Here's how the part is built. I have some questions about the finished solid (model axes, mm). A direction names the side the tool comes from. Give positions to 0.01 mm unless a question says otherwise; leave off trailing zeros. Order: outer loops, then holes, each group sorted by start corner. A loop starts at its lowest first (then second) coordinate and runs counter-clockwise, first axis right, second up. Notation, with made-up numbers: (-37.5, -31.75) -> (12.5, -31.75) arc R20 ccw to (12.5, -12.75) -> close; hole circle Ø8 at (6, -31.5). An arc over 180 degrees is marked (long way). Write each question's results on one line, items separated by ' | '. Start each with the question number.
Q1. Imagine slicing it at B-B, the plane z = 5.5. Please give me the cut outline in (x, y).
Q2. Imagine slicing it at A-A, the plane y = -28. Please give me the cut outline in (x, z), then the cut area to 3 significant figures.
Q3. I need wall thicknesses on line 1 along X through (y, z) = (-43, 24); line 2 along Z through (x, y) = (-29, -39); line 3 along Y through (x, z) = (-0.5, 44). Which ranges of each line are inside material? Lowest first, please. Write a range as [from, to].
Q4. Thinking about a two-plate mould opening in X: for faces 1 (the face through (35, 29, 30)), 2 (the face through (92.171, 0, 52)), 3 (the face through (53, 20, 70)), which applies, pulls with the +X half, pulls with the -X half, needs draft (parallel to the pull), parting line crosses it, or undercut?
Q5. I'm going to push flat-ended pins straight in: pin 1 (4 mm diameter, centred on x = 85, z = 60, fed in from -Y); pin 2 (9 mm diameter, centred on x = 84.5, y = 32.5, fed in from +Z); pin 3 (7.5 mm diameter, centred on y = -0.5, z = 53, fed in from -X). Where does each tip first touch, or does it pass through?
Q6. Imagine slicing it at C-C, the plane x = 135. Please give me the cut outline in (y, z).
Q7. For faces 4 (the face through (106.877, -29, 62)), 5 (the face through (106.877, 29, 62)), 6 (the face through (89, -29, 70)), 7 (the face through (122, 0, 48.198)), which set-ups out of +Z, -Z, +X, -X, +Y, -Y let a thin tool reach every point of the face, with its end or its side?
```python
from build123d import *

# Parameters (mm, degrees)
F1_DEPTH = 62.5
F0_W     = 14.7052842798
F0_H     = 15
F2_DEPTH = 37.5
F0_H_2   = 6.8016763031
F0_H_3   = 8.1983236969
F3_DEPTH = 20


with BuildPart() as f1:
    # F0 (on Front) → F1 (new body, symmetric)
    with BuildSketch(Plane.XZ):
        Polygon((-50, 25), (-50, -25), (50, -25), (50, 25), (35, 25), align=None)
    extrude(amount=F1_DEPTH, both=True)

    # F0 (on Front) → F2 (join, symmetric)
    with BuildSketch(Plane.XZ):
        with Locations((99.52410253, 62.5)):
            Rectangle(F0_W, F0_H)
        with BuildLine():
            Line((35, 25), (50, 25))
            Line((50, 25), (50, 35))
            ThreePointArc((50, 35), (55.8578643763, 49.1421356237), (70, 55))
            Line((70, 55), (92.1714603901, 55))
            Line((92.1714603901, 55), (92.1714603901, 70))
            Line((92.1714603901, 70), (70, 70))
            ThreePointArc((70, 70), (45.2512626585, 59.7487373415), (35, 35))
            Line((35, 35), (35, 25))
        make_face()
    extrude(amount=F2_DEPTH, both=True)

    # F0 (on Front) → F3 (join, symmetric)
    with BuildSketch(Plane.XZ):
        with BuildLine():
            add(Edge.make_bspline(
                [(-50, 25), (-4.2251776904, 70.7326084375), (24.2556538433, 74.8012959957), (92.1714603901, 78.1983236969)],
                knots=[0, 0, 0, 0, 151.7985039241, 151.7985039241, 151.7985039241, 151.7985039241], degree=3))
            Line((-50, 25), (35, 25))
            Line((35, 25), (35, 35))
            ThreePointArc((35, 35), (45.2512626585, 59.7487373415), (70, 70))
            Line((70, 70), (92.1714603901, 70))
            Line((92.1714603901, 70), (92.1714603901, 78.1983236969))
        make_face()
        Polygon((106.8767446699, 48.1983236969), (137.2651457787, 48.1983236969), (152.1714603901, 48.1983236969), (152.1714603901, 78.1983236969), (127.8208345175, 78.1983236969), (106.8767446699, 78.1983236969), (106.8767446699, 70), (106.8767446699, 55), align=None)
        with Locations((99.52410253, 51.5991618484)):
            Rectangle(F0_W, F0_H_2)
        with Locations((99.52410253, 74.0991618484)):
            Rectangle(F0_W, F0_H_3)
    extrude(amount=F3_DEPTH, both=True)


solid = f1.part
```
Geometry check:
1) outline: (-50, -62.5) -> (50, -62.5) -> (50, 62.5) -> (-50, 62.5) -> close
2) outline: (-50, -25) -> (50, -25) -> (50, 35) arc R20 cw to (70, 55) -> (106.88, 55) -> (106.88, 70) -> (70, 70) arc R35 ccw to (35, 35) -> (35, 25) -> (-50, 25) -> close | area: 6,350 mm²
3) line 1: [-50, 50] | line 2: [-25, 25] | line 3: [-20, 20]
4) face 1: pulls with the -X half | face 2: undercut | face 3: needs draft
5) pin 1: y = -37.5 | pin 2: z = 70 | pin 3: x = -22.14
6) outline: (-20, 48.2) -> (20, 48.2) -> (20, 78.2) -> (-20, 78.2) -> close
7) face 4: +Z, -Z, +X, -Y | face 5: +Z, -Z, +X, +Y | face 6: +Z, +X, -X, -Y | face 7: -Z, +X, +Y, -Y
